Part model, mm, in its own coordinate system. Face numbers are marked on the shaded views. Coordinates: 2 decimals unless noted, no trailing zeros. Write each loop counter-clockwise with the first axis right and the second up, starting at its lowest first coordinate (ties: lowest second). Pieces come first, ordered by that corner, then holes. Notation, with made-up numbers: (33.5, 87) -> (88.5, 87) arc R17 cw to (88.5, 119) -> close; hole circle Ø1 at (86.25, 34). An arc over 180 degrees is marked (long way). One line per question, with ' | ' between items. Start each with the question number.
Item 1: Saw through at A-A (z = -39.5). List the corners of the cut face in (x, y), and give its area (3 significant figures).
Item 2: Saw through at B-B (x = -72). List the corners of the cut face in (y, z).
Item 3: Pin check, flat tips, straight feed: pin 1 (0.5 mm diameter, centred on y = 0.5, z = 23.5, fed in from +X); pin 2 (6 mm diameter, centred on x = 105.5, z = -16.5, fed in from +Y); pin 3 (0.5 mm diameter, centred on x = 133, y = 0.5, fed in from -Z); pin 4 (1.1 mm diameter, centred on y = 0.5, z = 22, fed in from -X). Stop position of each tip, or through.
Item 4: Two-plate mould, pull along X, no slides. Class the marked faces 1 and 2: pulls with the +X half, pulls with the -X half, needs draft (parallel to the pull), parting line crosses it, or undercut.
Item 5: Probe probe 1 along X at (y, z) = (0.5, -51.5); probe 2 along X at (y, z) = (-2, -5); probe 3 along Y at (x, z) = (-10.5, -19). List the from-to ranges inside material, lowest first. Write a range as [from, to].
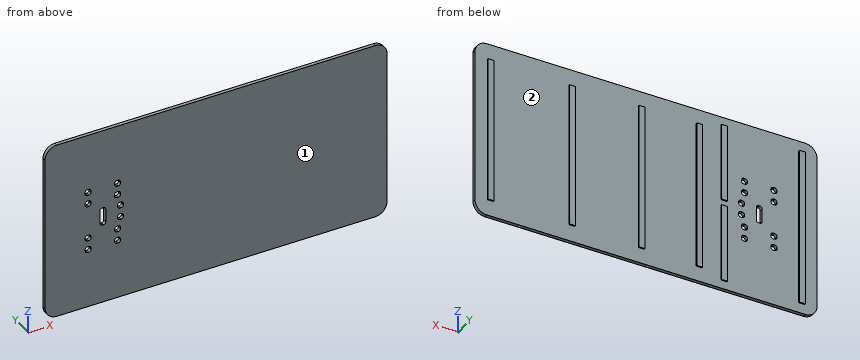
from build123d import *

# Parameters (mm, degrees)
SKETCH2_W                = 5
SKETCH2_H                = 133
ELEMENTGEOMETRY_DEPTH    = 1
SKETCH2_H_2              = 65.435
ELEMENTGEOMETRY_2_DEPTH  = 1
ELEMENTGEOMETRY_3_DEPTH  = 1
SKETCH2_H_3              = 125
ELEMENTGEOMETRY_4_DEPTH  = 1
SKETCH2_H_4              = 124
ELEMENTGEOMETRY_5_DEPTH  = 1
SKETCH2_H_5              = 123
ELEMENTGEOMETRY_6_DEPTH  = 1
SKETCH2_H_6              = 122
ELEMENTGEOMETRY_7_DEPTH  = 1
SKETCH5_W                = 290
SKETCH5_H                = 150
BOARDGEOMETRY_DEPTH      = 3
CABLECUTOUT_REACH        = 165.276
SKETCH7_W                = 5
SKETCH7_H                = 5
SKETCH7_H_2              = 15
MOUNTINGHOLES_DEPTH      = 164.275840221
MOUNTINGHOLES_DEPTH_BACK = 164.275840221
SKETCH8_W                = 5
SKETCH8_H                = 5
BOARDFILLET_R            = 10
MOUNTINGHOLEFILLET_R     = 2


with BuildPart() as part:
    # Sketch2 → ElementGeometry (new body)
    with BuildSketch(Plane(origin=(0, 0, 0), x_dir=(1, 0, 0), z_dir=(0, 1, 0))):
        with Locations((-132, 0)):
            Rectangle(SKETCH2_W, SKETCH2_H)
    extrude(amount=ELEMENTGEOMETRY_DEPTH)



with BuildPart() as body_2:
    # Sketch2 → ElementGeometry 2 (new body)
    with BuildSketch(Plane(origin=(0, 0, 0), x_dir=(1, 0, 0), z_dir=(0, 1, 0))):
        with Locations((-66, 35.2175)):
            Rectangle(SKETCH2_W, SKETCH2_H_2)
    extrude(amount=ELEMENTGEOMETRY_2_DEPTH)


with BuildPart() as body_3:
    # Sketch2 → ElementGeometry 3 (new body)
    with BuildSketch(Plane(origin=(0, 0, 0), x_dir=(1, 0, 0), z_dir=(0, 1, 0))):
        with Locations((-66, -35.2175)):
            Rectangle(SKETCH2_W, SKETCH2_H_2)
    extrude(amount=ELEMENTGEOMETRY_3_DEPTH)


with BuildPart() as body_4:
    # Sketch2 → ElementGeometry 4 (new body)
    with BuildSketch(Plane(origin=(0, 0, 0), x_dir=(1, 0, 0), z_dir=(0, 1, 0))):
        with Locations((-45, 0)):
            Rectangle(SKETCH2_W, SKETCH2_H_3)
    extrude(amount=ELEMENTGEOMETRY_4_DEPTH)


with BuildPart() as body_5:
    # Sketch2 → ElementGeometry 5 (new body)
    with BuildSketch(Plane(origin=(0, 0, 0), x_dir=(1, 0, 0), z_dir=(0, 1, 0))):
        with Locations((4, 0)):
            Rectangle(SKETCH2_W, SKETCH2_H_4)
    extrude(amount=ELEMENTGEOMETRY_5_DEPTH)


with BuildPart() as body_6:
    # Sketch2 → ElementGeometry 6 (new body)
    with BuildSketch(Plane(origin=(0, 0, 0), x_dir=(1, 0, 0), z_dir=(0, 1, 0))):
        with Locations((132, 0)):
            Rectangle(SKETCH2_W, SKETCH2_H_5)
    extrude(amount=ELEMENTGEOMETRY_6_DEPTH)


with BuildPart() as body_7:
    # Sketch2 → ElementGeometry 7 (new body)
    with BuildSketch(Plane(origin=(0, 0, 0), x_dir=(1, 0, 0), z_dir=(0, 1, 0))):
        with Locations((63, 0)):
            Rectangle(SKETCH2_W, SKETCH2_H_6)
    extrude(amount=ELEMENTGEOMETRY_7_DEPTH)


with BuildPart() as part_1:
    add(part.part)

    add(body_2.part)  # BoardGeometry merges body 2

    add(body_3.part)  # BoardGeometry merges body 3

    add(body_4.part)  # BoardGeometry merges body 4

    add(body_5.part)  # BoardGeometry merges body 5

    add(body_6.part)  # BoardGeometry merges body 6

    add(body_7.part)  # BoardGeometry merges body 7
    # Sketch5 → BoardGeometry (add)
    with BuildSketch(Plane(origin=(0, 0, 0), x_dir=(1, 0, 0), z_dir=(0, 1, 0))):
        Rectangle(SKETCH5_W, SKETCH5_H)
    extrude(amount=-BOARDGEOMETRY_DEPTH)

    # Sketch7 → CableCutout (cut, up to next)
    with BuildSketch(Plane(origin=(0, 0, 0), x_dir=(1, 0, 0), z_dir=(0, 1, 0)), mode=Mode.PRIVATE) as cablecutout_sk1:
        with Locations((-81, -5)):
            Rectangle(SKETCH7_W, SKETCH7_H)
    cablecutout_tool1 = extrude(cablecutout_sk1.sketch, amount=-CABLECUTOUT_REACH, mode=Mode.PRIVATE) & part_1.part
    # Sketch7 → CableCutout (cut, up to next)
    with BuildSketch(Plane(origin=(0, 0, 0), x_dir=(1, 0, 0), z_dir=(0, 1, 0)), mode=Mode.PRIVATE) as cablecutout_sk2:
        with Locations((-81, 5)):
            Rectangle(SKETCH7_W, SKETCH7_H)
    cablecutout_tool2 = extrude(cablecutout_sk2.sketch, amount=-CABLECUTOUT_REACH, mode=Mode.PRIVATE) & part_1.part
    # Sketch7 → CableCutout (cut, up to next)
    with BuildSketch(Plane(origin=(0, 0, 0), x_dir=(1, 0, 0), z_dir=(0, 1, 0)), mode=Mode.PRIVATE) as cablecutout_sk3:
        with Locations((-96, 0)):
            Rectangle(SKETCH7_W, SKETCH7_H_2)
    cablecutout_tool3 = extrude(cablecutout_sk3.sketch, amount=-CABLECUTOUT_REACH, mode=Mode.PRIVATE) & part_1.part
    add(cablecutout_tool1.solids().sort_by_distance((-81, 0, 5))[0], mode=Mode.SUBTRACT)
    add(cablecutout_tool2.solids().sort_by_distance((-81, 0, -5))[0], mode=Mode.SUBTRACT)
    add(cablecutout_tool3.solids().sort_by_distance((-96, 0, 0))[0], mode=Mode.SUBTRACT)

    # Sketch8 → MountingHoles (cut, two sides: drawn at the far end of the back side and taken through both)
    with BuildSketch(Plane(origin=(0, 0, 0), x_dir=(1, 0, 0), z_dir=(0, 1, 0)).offset(-MOUNTINGHOLES_DEPTH_BACK)):
        with Locations((-108.5, 15)):
            Rectangle(SKETCH8_W, SKETCH8_H)
        with Locations((-83.5, 15)):
            Rectangle(SKETCH8_W, SKETCH8_H)
        with Locations((-83.5, -15)):
            Rectangle(SKETCH8_W, SKETCH8_H)
        with Locations((-108.5, -15)):
            Rectangle(SKETCH8_W, SKETCH8_H)
        with Locations((-83.5, -25)):
            Rectangle(SKETCH8_W, SKETCH8_H)
        with Locations((-108.5, -25)):
            Rectangle(SKETCH8_W, SKETCH8_H)
        with Locations((-83.5, 25)):
            Rectangle(SKETCH8_W, SKETCH8_H)
        with Locations((-108.5, 25)):
            Rectangle(SKETCH8_W, SKETCH8_H)
    extrude(amount=MOUNTINGHOLES_DEPTH + MOUNTINGHOLES_DEPTH_BACK, mode=Mode.SUBTRACT)

    # BoardFillet
    boardfillet_edges = [part_1.edges().sort_by_distance(p)[0] for p in [
        (-145, -1.5, -75),
        (145, -1.5, -75),
        (145, -1.5, 75),
        (-145, -1.5, 75),
    ]]
    fillet(boardfillet_edges, radius=BOARDFILLET_R)

    # MountingHoleFillet
    mountingholefillet_edges = [part_1.edges().sort_by_distance(p)[0] for p in [
        (-78.5, -1.5, -2.5),
        (-83.5, -1.5, -2.5),
        (-83.5, -1.5, -7.5),
        (-78.5, -1.5, -7.5),
        (-78.5, -1.5, 2.5),
        (-78.5, -1.5, 7.5),
        (-83.5, -1.5, 7.5),
        (-83.5, -1.5, 2.5),
        (-111, -1.5, 12.5),
        (-106, -1.5, 12.5),
        (-106, -1.5, 17.5),
        (-111, -1.5, 17.5),
        (-86, -1.5, 12.5),
        (-81, -1.5, 12.5),
        (-81, -1.5, 17.5),
        (-86, -1.5, 17.5),
        (-106, -1.5, 22.5),
        (-106, -1.5, 27.5),
        (-111, -1.5, 27.5),
        (-111, -1.5, 22.5),
        (-86, -1.5, -17.5),
        (-81, -1.5, -17.5),
        (-81, -1.5, -12.5),
        (-86, -1.5, -12.5),
        (-81, -1.5, 22.5),
        (-81, -1.5, 27.5),
        (-86, -1.5, 27.5),
        (-86, -1.5, 22.5),
        (-81, -1.5, -27.5),
        (-81, -1.5, -22.5),
        (-86, -1.5, -22.5),
        (-86, -1.5, -27.5),
        (-106, -1.5, -22.5),
        (-111, -1.5, -22.5),
        (-111, -1.5, -27.5),
        (-106, -1.5, -27.5),
        (-106, -1.5, -17.5),
        (-106, -1.5, -12.5),
        (-111, -1.5, -12.5),
        (-111, -1.5, -17.5),
        (-93.5, -1.5, -7.5),
        (-93.5, -1.5, 7.5),
        (-98.5, -1.5, 7.5),
        (-98.5, -1.5, -7.5),
    ]]
    fillet(mountingholefillet_edges, radius=MOUNTINGHOLEFILLET_R)


solid = part_1.part
From the geometry:
1) outline: (-145, -3) -> (145, -3) -> (145, 0) -> (134.5, 0) -> (134.5, 1) -> (129.5, 1) -> (129.5, 0) -> (65.5, 0) -> (65.5, 1) -> (60.5, 1) -> (60.5, 0) -> (6.5, 0) -> (6.5, 1) -> (1.5, 1) -> (1.5, 0) -> (-42.5, 0) -> (-42.5, 1) -> (-47.5, 1) -> (-47.5, 0) -> (-63.5, 0) -> (-63.5, 1) -> (-68.5, 1) -> (-68.5, 0) -> (-129.5, 0) -> (-129.5, 1) -> (-134.5, 1) -> (-134.5, 0) -> (-145, 0) -> close | area: 900 mm2
2) outline: (-3, -75) -> (0, -75) -> (0, 75) -> (-3, 75) -> close
3) pin 1: x = 134.5 | pin 2: y = 0 | pin 3: z = -61.5 | pin 4: x = -145
4) face 1: needs draft | face 2: undercut
5) probe 1: [-134.5, -129.5], [-68.5, -63.5], [-47.5, -42.5], [1.5, 6.5], [60.5, 65.5], [129.5, 134.5] | probe 2: [-145, -98.5], [-93.5, -83.5], [-78.5, 145] | probe 3: [-3, 0]
